Design review of the part shown in the three views and the two pictorial views. Dimensions are in mm from the part's minimum x, y and z. A direction names the side the tool comes from. Coordinates: 2 decimals unless noted, no trailing zeros. Loops run counter-clockwise (first coordinate to the right, second up) from the corner with the lowest first, then second, coordinate; pieces in that order, holes last.
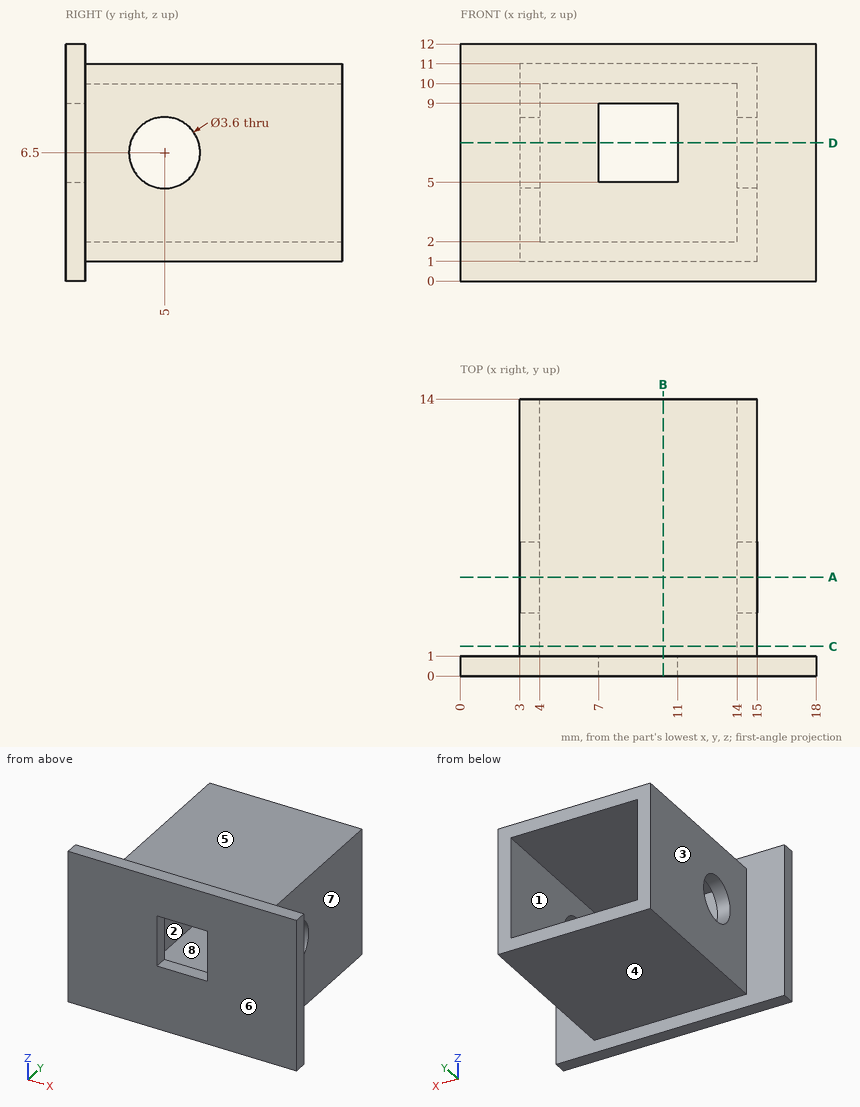
Q1. Machinability: for the marked faces 5, 6, 7 and 8, which of the approach directions +Z, -Z, +X, -X, +Y, -Y give a long, thin tool a straight path to every point of the face, cutting with its end or side? Answer none if there is none.
Q2. The part is to be moulded in two halves that separate along X. For the marked faces 1, 2, 3 and 4, say which applies: +X half, -X half, draft (parallel to the pull), parting line (faces both ways), or undercut.
Q3. Consider section D-D (z = 7). State the section outline as (x, y) points.
Q4. Wall thickness on probe 1 along X at (y, z) = (9.75, 4); probe 2 along Y at (x, z) = (14.2, 6.5); probe 3 along Z at (x, y) = (11.5, 2.75): over which ranges is each line inside the solid? List them lowest first.
Q5. Consider section B-B (x = 10.25). State the section outline as (y, z) points.
Q6. Consider section A-A (y = 5). State the section outline as (x, z) points.
Q7. Consider section C-C (y = 1.5). State the section outline as (x, z) points, then the cut area to 3 significant figures.
Q8. For pin 1 Ø6 at (x, y) = (8, 10) entering from +Z; pin 2 Ø4 at (y, z) = (5, 6.5) entering from -X; pin 3 Ø3 at (x, y) = (13, 9.5) entering from -Z, all flat-tipped, find the tip position at first contact; note any pin that passes through.
Model answer:
1. face 5: +Z, +X, -X, +Y
1. face 6: +Z, -Z, +X, -X, -Y
1. face 7: +Z, -Z, +X, +Y
1. face 8: +Y
2. face 1: undercut
2. face 2: undercut
2. face 3: -X half
2. face 4: draft
3. outline: (0, 0) - (7, 0) - (7, 1) - (4, 1) - (4, 3.27) - (3, 3.27) - (3, 1) - (0, 1) - close; (3, 6.73) - (4, 6.73) - (4, 14) - (3, 14) - close; (11, 0) - (18, 0) - (18, 1) - (15, 1) - (15, 3.27) - (14, 3.27) - (14, 1) - (11, 1) - close; (14, 6.73) - (15, 6.73) - (15, 14) - (14, 14) - close
4. probe 1: x = 3 to 4, 14 to 15
4. probe 2: y = 0 to 3.2, 6.8 to 14
4. probe 3: z = 1 to 2, 10 to 11
5. outline: (0, 0) - (1, 0) - (1, 1) - (14, 1) - (14, 2) - (1, 2) - (1, 5) - (0, 5) - close; (0, 9) - (1, 9) - (1, 10) - (14, 10) - (14, 11) - (1, 11) - (1, 12) - (0, 12) - close
6. outline: (3, 1) - (15, 1) - (15, 4.7) - (14, 4.7) - (14, 2) - (4, 2) - (4, 4.7) - (3, 4.7) - close; (3, 8.3) - (4, 8.3) - (4, 10) - (14, 10) - (14, 8.3) - (15, 8.3) - (15, 11) - (3, 11) - close
7. outline: (3, 1) - (15, 1) - (15, 11) - (3, 11) - close; hole (4, 2) - (14, 2) - (14, 10) - (4, 10) - close
7. area: 40.0 mm2
8. pin 1: stops at z = 11
8. pin 2: stops at x = 3
8. pin 3: stops at z = 1
